The listing builds one solid part. Answer for the finished solid, in the listing's coordinates (mm). Give positions to 0.01 mm unless a question says otherwise; leave off trailing zeros. Order: outer loops, then holes, each group sorted by start corner. A loop starts at its lowest first (then second) coordinate and runs counter-clockwise, first axis right, second up.
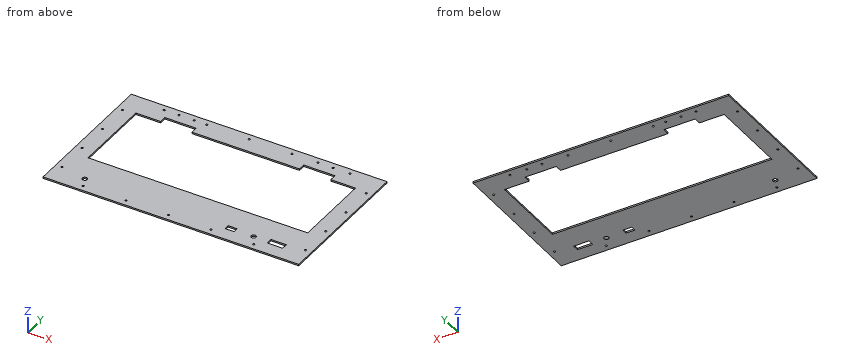
```python
from build123d import *

# Parameters (mm, degrees)
SKETCH1_W           = 533.4
SKETCH1_H           = 304.8
BOSS_EXTRUDE1_DEPTH = 3.175
SKETCH5_R           = 2.032
CUT_EXTRUDE4_DEPTH  = 4.175
SKETCH6_R           = 2.032
CUT_EXTRUDE5_DEPTH  = 3.175
SKETCH7_R           = 2.032
CUT_EXTRUDE6_DEPTH  = 4.175
SKETCH8_W           = 458.193815808
SKETCH8_H           = 165.1
SKETCH8_W_2         = 65.278
SKETCH8_H_2         = 14.478
CUT_EXTRUDE7_DEPTH  = 4.175
SKETCH9_R           = 4.953
SKETCH9_W           = 32.258
SKETCH9_H           = 12.954
SKETCH9_W_2         = 18.542
SKETCH9_H_2         = 10.668
CUT_EXTRUDE8_DEPTH  = 4.175


with BuildPart() as part:
    # Sketch1 → Boss-Extrude1 (new body)
    with BuildSketch(Plane.XY):
        with Locations((266.7, 152.4)):
            Rectangle(SKETCH1_W, SKETCH1_H)
    extrude(amount=BOSS_EXTRUDE1_DEPTH)

    # Sketch5 → Cut-Extrude4 (cut, through all)
    with BuildSketch(Plane.XY.offset(3.175)):
        with Locations((76.2, 12.7)):
            Circle(SKETCH5_R)
        with Locations((165.1, 12.7)):
            Circle(SKETCH5_R)
        with Locations((254, 12.7)):
            Circle(SKETCH5_R)
        with Locations((342.9, 12.7)):
            Circle(SKETCH5_R)
        with Locations((431.8, 12.7)):
            Circle(SKETCH5_R)
        with Locations((342.9, 292.1)):
            Circle(SKETCH5_R)
        with Locations((254, 292.1)):
            Circle(SKETCH5_R)
        with Locations((165.1, 292.1)):
            Circle(SKETCH5_R)
        with Locations((76.2, 292.1)):
            Circle(SKETCH5_R)
        with Locations((463.719540129, 292.1)):
            Circle(SKETCH5_R)
    extrude(amount=-CUT_EXTRUDE4_DEPTH, mode=Mode.SUBTRACT)

    # Sketch6 → Cut-Extrude5 (cut)
    with BuildSketch(Plane.XY.offset(3.175)):
        with Locations((12.7, 254)):
            Circle(SKETCH6_R)
        with Locations((12.7, 184.15)):
            Circle(SKETCH6_R)
        with Locations((12.7, 114.3)):
            Circle(SKETCH6_R)
        with Locations((12.7, 44.45)):
            Circle(SKETCH6_R)
        with Locations((520.7, 44.45)):
            Circle(SKETCH6_R)
        with Locations((520.7, 114.3)):
            Circle(SKETCH6_R)
        with Locations((520.7, 184.15)):
            Circle(SKETCH6_R)
        with Locations((520.7, 254)):
            Circle(SKETCH6_R)
    extrude(amount=-CUT_EXTRUDE5_DEPTH, mode=Mode.SUBTRACT)

    # Sketch7 → Cut-Extrude6 (cut, through all)
    with BuildSketch(Plane(origin=(0, 0, 0), x_dir=(-1, 0, 0), z_dir=(0, 0, -1))):
        with Locations((-138.857978908, 292.182920205)):
            Circle(SKETCH7_R)
        with Locations((-107.107978908, 292.182920205)):
            Circle(SKETCH7_R)
        with Locations((-428.774184192, 292.182920205)):
            Circle(SKETCH7_R)
        with Locations((-397.024184192, 292.182920205)):
            Circle(SKETCH7_R)
    extrude(amount=-CUT_EXTRUDE6_DEPTH, mode=Mode.SUBTRACT)

    # Sketch8 → Cut-Extrude7 (cut, through all)
    with BuildSketch(Plane.XY.offset(3.175)):
        with Locations((266.711092096, 175.755983959)):
            Rectangle(SKETCH8_W, SKETCH8_H)
        with Locations((121.815184192, 265.544983959)):
            Rectangle(SKETCH8_W_2, SKETCH8_H_2)
        with Locations((411.607, 265.544983959)):
            Rectangle(SKETCH8_W_2, SKETCH8_H_2)
    extrude(amount=-CUT_EXTRUDE7_DEPTH, mode=Mode.SUBTRACT)

    # Sketch9 → Cut-Extrude8 (cut, through all)
    with BuildSketch(Plane.XY.offset(3.175)):
        with Locations((419.1, 33.528)):
            Circle(SKETCH9_R)
        with Locations((66.977757166, 33.528)):
            Circle(SKETCH9_R)
        with Locations((466.471, 35.052)):
            Rectangle(SKETCH9_W, SKETCH9_H)
        with Locations((371.729, 33.909)):
            Rectangle(SKETCH9_W_2, SKETCH9_H_2)
    extrude(amount=-CUT_EXTRUDE8_DEPTH, mode=Mode.SUBTRACT)


solid = part.part
```
1) Find section C-C (x = 419.1). Write down the section's boundary in (y, z) (3 decimals), then the cut area to 3 significant figures.
Geometry says:
outline: (0, 0) - (28.575, 0) - (28.575, 3.175) - (0, 3.175) - close; (38.481, 0) - (93.206, 0) - (93.206, 3.175) - (38.481, 3.175) - close; (272.784, 0) - (304.8, 0) - (304.8, 3.175) - (272.784, 3.175) - close
area: 366 mm2
2) Straight lines are drawn through the part: probe 1 along X at (y, z) = (263, 2.2); probe 2 along Y at (x, z) = (165.1, 1.55); probe 3 along X at (y, z) = (184.15, 0.6). For each, find the intervals that lie inside material, in ascending order.
Geometry says:
probe 1: x = 0 to 89.18, 154.45 to 378.97, 444.25 to 533.4
probe 2: y = 0 to 10.67, 14.73 to 93.21, 258.31 to 290.07, 294.13 to 304.8
probe 3: x = 0 to 10.67, 14.73 to 37.61, 495.81 to 518.67, 522.73 to 533.4
3) Find section D-D (z = 2.15). Count the separate pieces of the cut face and the enclosed holes in it, then the cut area to 3 significant figures.
Geometry says:
separate pieces: 1
enclosed holes: 27
area: 84,000 mm2
4) Find section B-B (y = 238). Write down the section's boundary in (x, z) (3 decimals), then the cut area to 3 significant figures.
Geometry says:
outline: (0, 0) - (37.614, 0) - (37.614, 3.175) - (0, 3.175) - close; (495.808, 0) - (533.4, 0) - (533.4, 3.175) - (495.808, 3.175) - close
area: 239 mm2
5) Find section A-A (x = 197). Write down the section's boundary in (y, z) (3 decimals), then the cut area to 3 significant figures.
Geometry says:
outline: (0, 0) - (93.206, 0) - (93.206, 3.175) - (0, 3.175) - close; (258.306, 0) - (304.8, 0) - (304.8, 3.175) - (258.306, 3.175) - close
area: 444 mm2
